Geometry: final body of the model. Coordinates: model frame, mm. A direction names the side the tool comes from. Round coordinates to 2 decimals unless told otherwise and drop trailing zeros. Loops run counter-clockwise (first coordinate to the right, second up) from the corner with the lowest first, then second, coordinate; pieces in that order, holes last. Notation, with made-up numbers: (47.5, -37.75) - (80.5, -37.75) arc R12 cw to (80.5, -24.75) - close; hole circle Ø8 at (17, 6.25). An arc over 180 degrees is marked (long way). Return JSON: item names as keys, results as strings. Group by question number.
1. Section A-A on x = 27.46. Return loops of the section in (y, z).
2. Material intervals for probe 1 along X at (y, z) = (-3.5, 9); probe 2 along Y at (x, z) = (27.46, 4.5); probe 3 along X at (y, z) = (-22, 7.5), sorted ascending.
3. Section D-D on z = 2.75. Return loops of the section in (x, y).
4. Draft query along X for faces 3 (the face through (-35, 0, 5)), 4 (the face through (0, 0, 0)), 5 (the face through (23.77, -24.07, 4.93)). Return one class per face: +X half, -X half, draft (parallel to the pull), parting line (faces both ways), or undercut.
5. Set-up query: faces 1 (the face through (0, -35, 5)), 2 (the face through (22.86, 0, 8)). Return all of +Z, -Z, +X, -X, +Y, -Y with unobstructed straight access to the full face (end or side cutting, diameter ignored); none if empty.
6. First-contact query: pin 1 Ø9 at (x, y) = (27.46, -27.46) entering from +Z. Flat tip, straight axial feed; report the tip coordinate or a pass-through.
7. Section B-B on x = 8.5. Return loops of the section in (y, z), and give its area (3 significant figures).
from build123d import *

# Parameters (mm, degrees)
F0_W     = 70
F0_H     = 70
F0_R     = 5.0038
F0_R_2   = 5
F1_DEPTH = 10
F2_W     = 45.72
F2_H     = 45.72
F2_W_2   = 35.56
F2_H_2   = 35.56
F3_DEPTH = 5


with BuildPart() as f1:
    # F0 (on Top) → F1 (new body)
    with BuildSketch(Plane.XY):
        Rectangle(F0_W, F0_H)
        with Locations((-27.4562, -27.4562)):
            Circle(F0_R, mode=Mode.SUBTRACT)
        with Locations((27.4562, -27.4562)):
            Circle(F0_R, mode=Mode.SUBTRACT)
        with Locations((-27.4562, 27.4562)):
            Circle(F0_R, mode=Mode.SUBTRACT)
        with Locations((27.46, 27.46)):
            Circle(F0_R_2, mode=Mode.SUBTRACT)
    extrude(amount=F1_DEPTH)

    # F2 (on face) → F3 (cut)
    with BuildSketch(Plane.XY.offset(10)):
        Rectangle(F2_W, F2_H)
        Rectangle(F2_W_2, F2_H_2, mode=Mode.SUBTRACT)
    extrude(amount=-F3_DEPTH, mode=Mode.SUBTRACT)


solid = f1.part
Taken from the geometry:
{
 "1": {"outline": "(-35, 0) - (-32.46, 0) - (-32.46, 10) - (-35, 10) - close; (-22.45, 0) - (22.46, 0) - (22.46, 10) - (-22.45, 10) - close; (32.46, 0) - (35, 0) - (35, 10) - (32.46, 10) - close"},
 "2": {"probe 1": "-35 to -22.86, -17.78 to 17.78, 22.86 to 35", "probe 2": "-35 to -32.46, -22.45 to 22.46, 32.46 to 35", "probe 3": "-35 to -22.86, 22.86 to 35"},
 "3": {"outline": "(-35, -35) - (35, -35) - (35, 35) - (-35, 35) - close; hole circle Ø10.01 at (-27.46, -27.46); hole circle Ø10.01 at (-27.46, 27.46); hole circle Ø10.01 at (27.46, -27.46); hole circle Ø10 at (27.46, 27.46)"},
 "4": {"face 3": "-X half", "face 4": "draft", "face 5": "undercut"},
 "5": {"face 1": "+Z, -Z, +X, -X, -Y", "face 2": "+Z"},
 "6": {"pin 1": "through"},
 "7": {"outline": "(-35, 0) - (35, 0) - (35, 10) - (22.86, 10) - (22.86, 5) - (17.78, 5) - (17.78, 10) - (-17.78, 10) - (-17.78, 5) - (-22.86, 5) - (-22.86, 10) - (-35, 10) - close", "area": "649 mm2"}
}
